```python
from build123d import *

# Parameters (mm, degrees)
F0_R     = 20.8
F0_R_2   = 3.5
F1_DEPTH = 1.2
F2_R     = 20.8
F2_R_2   = 3.5
F3_DEPTH = 3
F4_R     = 20.8
F4_R_2   = 1.5
F5_DEPTH = 3.9
F6_R     = 2.65
F7_DEPTH = 1.2


with BuildPart() as f1:
    # F0 (on Top) → F1 (new body)
    with BuildSketch(Plane.XY):
        with Locations((20.8, 20.8)):
            Circle(F0_R)
        with Locations((5.8, 20.8)):
            Circle(F0_R_2, mode=Mode.SUBTRACT)
        with Locations((35.8, 20.8)):
            Circle(F0_R_2, mode=Mode.SUBTRACT)
    extrude(amount=F1_DEPTH)

    # F2 (on face) → F3 (join)
    with BuildSketch(Plane.XY.offset(1.2)):
        with Locations((20.8, 20.8)):
            Circle(F2_R)
        with BuildLine():
            ThreePointArc((39.073, 16.379879), (20.8, 2), (2.527, 16.379879))
            ThreePointArc((2.527, 16.379879), (11.3, 20.8), (2.527, 25.220121))
            ThreePointArc((2.527, 25.220121), (20.8, 39.6), (39.073, 25.220121))
            ThreePointArc((39.073, 25.220121), (30.3, 20.8), (39.073, 16.379879))
        make_face(mode=Mode.SUBTRACT)
        with Locations((5.8, 20.8)):
            Circle(F2_R_2, mode=Mode.SUBTRACT)
        with Locations((35.8, 20.8)):
            Circle(F2_R_2, mode=Mode.SUBTRACT)
    extrude(amount=F3_DEPTH)

    # F4 (on face) → F5 (join)
    with BuildSketch(Plane.XY.offset(4.2)):
        with Locations((20.8, 20.8)):
            Circle(F4_R)
        with BuildLine():
            ThreePointArc((39.073, 16.379879), (20.8, 2), (2.527, 16.379879))
            ThreePointArc((2.527, 16.379879), (11.3, 20.8), (2.527, 25.220121))
            ThreePointArc((2.527, 25.220121), (20.8, 39.6), (39.073, 25.220121))
            ThreePointArc((39.073, 25.220121), (30.3, 20.8), (39.073, 16.379879))
        make_face(mode=Mode.SUBTRACT)
        with Locations((5.8, 20.8)):
            Circle(F4_R_2, mode=Mode.SUBTRACT)
        with Locations((35.8, 20.8)):
            Circle(F4_R_2, mode=Mode.SUBTRACT)
    extrude(amount=F5_DEPTH)

    # F6 (on face) → F7 (cut, through all)
    with BuildSketch(Plane.XY.offset(1.2)):
        with Locations((14.304809, 24.55)):
            Circle(F6_R)
        with Locations((20.8, 28.3)):
            Circle(F6_R)
        with Locations((27.295191, 24.55)):
            Circle(F6_R)
        with Locations((27.295191, 17.05)):
            Circle(F6_R)
        with Locations((20.8, 13.3)):
            Circle(F6_R)
        with Locations((14.304809, 17.05)):
            Circle(F6_R)
    extrude(amount=-F7_DEPTH, mode=Mode.SUBTRACT)


solid = f1.part
```
Could you check a few things on this model? Use its own coordinates, in mm. A direction names the side the tool comes from. Coordinates: 2 decimals unless noted, no trailing zeros. Write each loop counter-clockwise with the first axis right and the second up, starting at its lowest first coordinate (ties: lowest second). Pieces come first, ordered by that corner, then holes. Notation, with made-up numbers: (49.5, -10) -> (74.5, -10) arc R13 cw to (74.5, 10) -> close; hole circle Ø6 at (39, 8). An arc over 180 degrees is marked (long way). One line per question, with ' | ' between items. Start each with the question number.
1. For faces 5 (the face through (3, 18.7, 2.1)), 6 (the face through (21, 21, 1.2)), 7 (the face through (20.23, 25.71, 0.61)), which set-ups out of +Z, -Z, +X, -X, +Y, -Y let a thin tool reach every point of the face, with its end or its side?
2. Please list where these lines run through material, in increasing order: line 1 along Y through (x, z) = (20.8, 0.3); line 2 along Y through (x, z) = (10, 2.25); line 3 along Y through (x, z) = (35.8, 6.7).
3. Will these pins go through, and if not, where does the flat tip stop? P1, Ø8.5, axis at x = 20.8, y = 28.3, coming from the -Z side; P2, Ø4, axis at y = 36.5, z = 2, coming from the -X side; P3, Ø3, axis at x = 32.5, z = 6, coming from the -Y side; P4, Ø3.5, axis at x = 4.5, y = 21.5, coming from the -Z side.
4. If we section it at B-B (z = 2.5): Please give me the cut outline in (x, y), and give its area (3 significant figures).
5. If we section it at C-C (y = 20.8): Please give me the cut outline in (x, z), and give its area (3 significant figures).
6. If we section it at D-D (y = 13.3): Please give me the cut outline in (x, z), and give its area (3 significant figures).
7. Thinking about a two-plate mould opening in X: for faces 1 (the face through (16.291, 0.495, 3.993)), 2 (the face through (21, 21, 0)), 3 (the face through (5.475, 19.336, 6.123)), 4 (the face through (33, 18.7, 2.1)), which applies, pulls with the +X half, pulls with the -X half, needs draft (parallel to the pull), parting line crosses it, or undercut?
8. If we section it at A-A (x = 20.8): Please give me the cut outline in (y, z), and give its area (3 significant figures).
Return value:
1) face 5: -Z | face 6: +Z | face 7: +Z, -Z
2) line 1: y = 0 to 10.65, 15.95 to 25.65, 30.95 to 41.6 | line 2: y = 3.02 to 5.41, 17.25 to 24.35, 36.19 to 38.58 | line 3: y = 6.39 to 9.47, 15.3 to 19.3, 22.3 to 26.3, 32.13 to 35.21
3) P1: stops at z = 0 | P2: stops at x = 5.15 | P3: stops at y = 2.67 | P4: stops at z = 4.2
4) outline: circle Ø41.6 at (20.8, 20.8); hole circle Ø7 at (5.8, 20.8); hole (2.53, 16.38) arc R18.8 ccw to (39.07, 16.38) arc R5.5 cw (long way) to (39.07, 25.22) arc R18.8 ccw to (2.53, 25.22) arc R5.5 cw (long way) to start; hole circle Ø7 at (35.8, 20.8) | area: 341 mm²
5) outline: (0, 0) -> (2.3, 0) -> (2.3, 4.2) -> (4.3, 4.2) -> (4.3, 8.1) -> (0, 8.1) -> close; (7.3, 4.2) -> (9.3, 4.2) -> (9.3, 0) -> (32.3, 0) -> (32.3, 4.2) -> (34.3, 4.2) -> (34.3, 8.1) -> (30.3, 8.1) -> (30.3, 1.2) -> (11.3, 1.2) -> (11.3, 8.1) -> (7.3, 8.1) -> close; (37.3, 4.2) -> (39.3, 4.2) -> (39.3, 0) -> (41.6, 0) -> (41.6, 8.1) -> (37.3, 8.1) -> close | area: 124 mm²
6) outline: (1.4, 0) -> (18.15, 0) -> (18.15, 1.2) -> (3.56, 1.2) -> (3.56, 8.1) -> (1.4, 8.1) -> close; (23.45, 0) -> (40.2, 0) -> (40.2, 8.1) -> (38.04, 8.1) -> (38.04, 1.2) -> (23.45, 1.2) -> close | area: 70.0 mm²
7) face 1: parting line crosses it | face 2: needs draft | face 3: undercut | face 4: undercut
8) outline: (0, 0) -> (10.65, 0) -> (10.65, 1.2) -> (2, 1.2) -> (2, 8.1) -> (0, 8.1) -> close; (15.95, 0) -> (25.65, 0) -> (25.65, 1.2) -> (15.95, 1.2) -> close; (30.95, 0) -> (41.6, 0) -> (41.6, 8.1) -> (39.6, 8.1) -> (39.6, 1.2) -> (30.95, 1.2) -> close | area: 64.8 mm²
